The figure shows three views and two pictorial views of one solid part (mm, origin at its lowest corner). Answer the questions. A direction names the side the tool comes from. Round coordinates to 2 decimals unless told otherwise and drop trailing zeros. Write each loop counter-clockwise with the first axis right and the second up, starting at its lowest first coordinate (ties: lowest second). Pieces come first, ordered by that corner, then holes.
Item 1: Find the intervals of material crossed by probe 1 along Z at (x, y) = (8, 13); probe 2 along X at (y, z) = (18, 17); probe 3 along Z at (x, y) = (5.5, 14.5), in increasing order.
Item 2: Each of these flat-tipped pins is pushed along its axis until it touches: pin 1 (3.5 mm diameter, centred on x = 36, z = 36, fed in from +Y); pin 2 (2 mm diameter, centred on x = 12.5, y = 33, fed in from -Z). Where does it stop, or does it pass through?
Item 3: Find section B-B on x = 36. Give the vertices of the cut face in (y, z), then the cut area to 3 significant figures.
Item 4: For a pull along X with two mould halves and no side action, classify the marked faces 1, 2, 3 and 4 as +X half, -X half, draft (parallel to the pull), parting line (faces both ways), or undercut.
Item 5: Find section A-A on z = 19. Give the vertices of the cut face in (x, y), then the cut area to 3 significant figures.
Item 6: A tool of negligible diameter and unlimited length cuts with its end or side. For the marked faces 5 and 6, from which of +Z, -Z, +X, -X, +Y, -Y can it reach the whole face along a straight path? Write none if from no direction.
Item 7: Find section C-C on y = 8.5. Give the vertices of the cut face in (x, z) (1 decimal).
Item 8: Find section D-D on z = 8. Give the vertices of the cut face in (x, y), then the cut area to 3 significant figures.
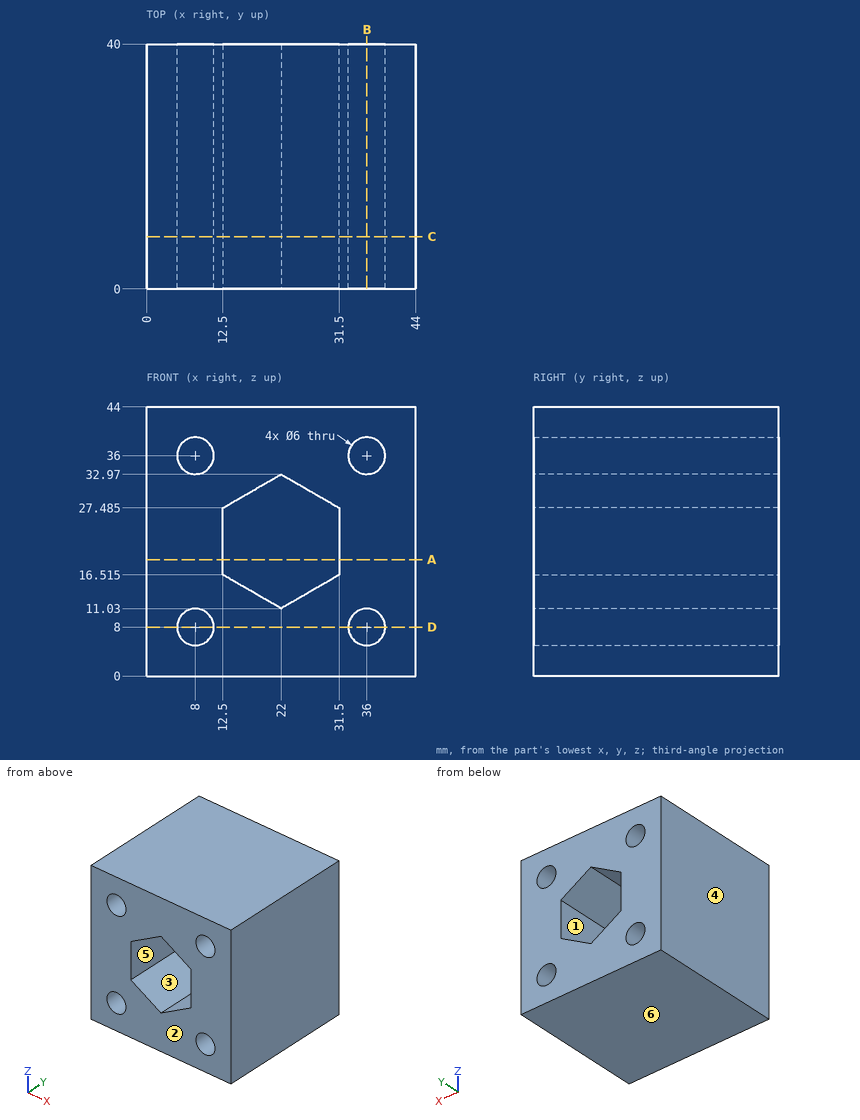
Check values:
1. probe 1: z = 0 to 5, 11 to 33, 39 to 44
1. probe 2: x = 0 to 12.5, 31.5 to 44
1. probe 3: z = 0 to 6.34, 9.66 to 34.34, 37.66 to 44
2. pin 1: passes through
2. pin 2: stops at z = 0
3. outline: (0, 0) - (40, 0) - (40, 5) - (0, 5) - close; (0, 11) - (40, 11) - (40, 33) - (0, 33) - close; (0, 39) - (40, 39) - (40, 44) - (0, 44) - close
3. area: 1,280 mm2
4. face 1: undercut
4. face 2: draft
4. face 3: undercut
4. face 4: -X half
5. outline: (0, 0) - (12.5, 0) - (12.5, 40) - (0, 40) - close; (31.5, 0) - (44, 0) - (44, 40) - (31.5, 40) - close
5. area: 1,000 mm2
6. face 5: +Y, -Y
6. face 6: -Z, +X, -X, +Y, -Y
7. outline: (0, 0) - (44, 0) - (44, 44) - (0, 44) - close; hole circle Ø6 at (8, 8); hole circle Ø6 at (8, 36); hole (12.5, 16.5) - (22, 11) - (31.5, 16.5) - (31.5, 27.5) - (22, 33) - (12.5, 27.5) - close; hole circle Ø6 at (36, 8); hole circle Ø6 at (36, 36)
8. outline: (0, 0) - (5, 0) - (5, 40) - (0, 40) - close; (11, 0) - (33, 0) - (33, 40) - (11, 40) - close; (39, 0) - (44, 0) - (44, 40) - (39, 40) - close
8. area: 1,280 mm2
